Geometry: final body of the model. Coordinates: model frame, mm. A direction names the side the tool comes from. Coordinates: 2 decimals unless noted, no trailing zeros. Order: outer loops, then holes, each group sorted by start corner. A loop starts at its lowest first (then second) coordinate and runs counter-clockwise, first axis right, second up. Notation, with made-up numbers: M -33,-27.75 L -24,-27.75 A33 cw -24,5.25 Z; hole C -30.5,-14.5 d9. An arc over 180 degrees is marked long. Use CSV: the item, a comma, the result in double quotes. Start each with the question number.
1. Section query D-D on x = -47. Return the cut outline in (y, z).
2. Pull-direction query (X, two-part tool) for faces 1 (the flat face through (-52.798, 14, -26)), 2 (the cylindrical face through (50.149, 20.585, -26.644)), 3 (the cylindrical face through (45.193, 50.176, -15.773)), 4 (the flat face through (29, 32, -43.7)); classes: pulls with the +X half, pulls with the -X half, needs draft (parallel to the pull), parting line crosses it, or undercut.
3. First-contact query: P1, Ø11, axis at x = -24.5, z = 6, coming from the +Y side; P2, Ø10, axis at x = -30, z = -40.5, coming from the +Y side; P3, Ø4, axis at y = 37.5, z = -12.5, coming from the -X side. Flat tips, straight axial feed; report the tip coordinate or a pass-through.
4. Section query A-A on z = -32.5. Return the cut outline in (x, y), and give its area (3 significant figures).
5. Material intervals for line 1 (Z direction, x = 41, y = 49); line 2 (Y direction, x = 47, z = -19.5); line 3 (X direction, y = 10.5, z = -34), sorted ascending.
6. Set-up query: faces 5 (the flat face through (-6, 5, -34)), 6 (the flat face through (-37.798, 23, -26)), 7 (the flat face through (-36, 0, 4)). Return all of +Z, -Z, +X, -X, +Y, -Y with unobstructed straight access to the full face (end or side cutting, diameter ignored); none if empty.
7. Section query C-C on y = 87.45. Return the cut outline in (x, z), and give its area (4 significant figures).
8. Section query B-B on x = 47. Return the cut outline in (y, z).
from build123d import *

# Parameters (mm, degrees)
SKETCH2_W                      = 90
SKETCH2_H                      = 30
BOSS_EXTRUDE1_DEPTH            = 184.15
SHELL1_T                       = 8
FILLET1_R                      = 10
CUT_EXTRUDE1_DEPTH             = 15
BOSS_EXTRUDE3_DEPTH            = 12.7
SKETCH19_W                     = 50.7
SKETCH19_H                     = 190.15
CUT_EXTRUDE3_DEPTH             = 160
CUT_EXTRUDE4_DEPTH             = 62.424750712
CUT_EXTRUDE5_DEPTH             = 83.99843372
CUT_EXTRUDE5_DEPTH_BACK        = 83.99843372
SKETCH21_W                     = 50.7
SKETCH21_H                     = 2
SKETCH22_W                     = 105.595917942
SKETCH22_H                     = 28.653888285
BOSS_EXTRUDE4_DEPTH            = 18
SKETCH25_W                     = 12
SKETCH25_H                     = 6
CUT_EXTRUDE7_DEPTH             = 69.833963067
BOSS_EXTRUDE6_DEPTH            = 10
SKETCH27_W                     = 12
SKETCH27_H                     = 8
BOSS_EXTRUDE7_DEPTH            = 26
SKETCH31_W                     = 15
SKETCH31_H                     = 38.653888285
BOSS_EXTRUDE8_DEPTH            = 10
F_5_16_0_3125_DIAMETER_HOLE2_D = 7.9375
SKETCH35_W                     = 52.9
SKETCH35_H                     = 70.8
BOSS_EXTRUDE9_DEPTH            = 15
F_5_5_5_5_DIAMETER_HOLE1_D     = 5.5
BOSS_EXTRUDE10_DEPTH           = 38.653888285
CUT_EXTRUDE8_DEPTH             = 20
CUT_EXTRUDE10_DEPTH            = 2
SKETCH43_W                     = 14.246111715
SKETCH43_H                     = 10
CUT_EXTRUDE11_DEPTH            = 157.542244125


with BuildPart() as part:
    # Sketch2 → Boss-Extrude1 (new body)
    with BuildSketch(Plane(origin=(0, 0, 0), x_dir=(1, 0, 0), z_dir=(0, 1, 0))):
        Rectangle(SKETCH2_W, SKETCH2_H)
    extrude(amount=BOSS_EXTRUDE1_DEPTH)

    # Shell1
    shell1_openings = [part.faces().sort_by_distance(p)[0] for p in [
        (0, 92.075, 15),
    ]]
    offset(amount=SHELL1_T, openings=shell1_openings, kind=Kind.INTERSECTION)

    # Fillet1
    # the kernel refuses this fillet: 10 mm, written as the material it adds along each edge
    with BuildSketch(Plane(origin=(-45, 0, -15), x_dir=(0, 1, 0), z_dir=(0, 0, 1)), Plane(origin=(45, 0, 15), x_dir=(0, 1, 0), z_dir=(0, 0, -1))) as fillet1_piece_1:
        with BuildLine():
            CenterArc((FILLET1_R, -FILLET1_R), FILLET1_R, 90, 90)
            Line((0, -FILLET1_R), (0, 0))
            Line((0, 0), (FILLET1_R, 0))
        make_face()
    extrude(amount=30)
    with BuildSketch(Plane(origin=(-45, 184.15, -15), x_dir=(0, -1, 0), z_dir=(0, 0, 1)), Plane(origin=(45, 184.15, 15), x_dir=(0, -1, 0), z_dir=(0, 0, -1))) as fillet1_piece_2:
        with BuildLine():
            CenterArc((FILLET1_R, FILLET1_R), FILLET1_R, 180, 90)
            Line((0, FILLET1_R), (0, 0))
            Line((0, 0), (FILLET1_R, 0))
        make_face()
    extrude(amount=30)
    # the kernel refuses this fillet: 10 mm, written as the material it takes off along each edge
    with BuildSketch(Plane(origin=(53, 192.15, 40), x_dir=(0, -1, 0), z_dir=(0, 0, -1)), Plane(origin=(-53, 192.15, -48), x_dir=(0, -1, 0), z_dir=(0, 0, 1)), Plane(origin=(-53, -8, -48), x_dir=(1, 0, 0), z_dir=(0, 0, 1))) as fillet1_2_piece_1:
        with BuildLine():
            CenterArc((FILLET1_R, FILLET1_R), FILLET1_R, 180, 90)
            Line((0, FILLET1_R), (0, 0))
            Line((0, 0), (FILLET1_R, 0))
        make_face()
    extrude(amount=88, mode=Mode.SUBTRACT)
    with BuildSketch(Plane(origin=(53, -8, 40), x_dir=(0, 1, 0), z_dir=(0, 0, -1))) as fillet1_2_piece_2:
        with BuildLine():
            CenterArc((FILLET1_R, -FILLET1_R), FILLET1_R, 90, 90)
            Line((0, -FILLET1_R), (0, 0))
            Line((0, 0), (FILLET1_R, 0))
        make_face()
    extrude(amount=88, mode=Mode.SUBTRACT)

    # Sketch3 → Cut-Extrude1 (cut)
    with BuildSketch(Plane.XZ.offset(8)):
        with BuildLine():
            Line((-21.5, 15), (21.5, 15))
            Line((21.5, 15), (21.5, 0))
            ThreePointArc((21.5, 0), (16.888679541, -5.139118926), (10.252551286, -7.046111715))
            Line((10.252551286, -7.046111715), (-10.252551286, -7.046111715))
            ThreePointArc((-10.252551286, -7.046111715), (-16.888679541, -5.139118926), (-21.5, 0))
            Line((-21.5, 0), (-21.5, 15))
        make_face()
    extrude(amount=-CUT_EXTRUDE1_DEPTH, mode=Mode.SUBTRACT)

    # Sketch16 → Boss-Extrude3 (add)
    with BuildSketch(Plane(origin=(0, 0, -23), x_dir=(-1, 0, 0), z_dir=(0, 0, -1))):
        with BuildLine():
            Line((-53, 182.15), (-53, 2))
            ThreePointArc((-53, 2), (-50.071067812, -5.071067812), (-43, -8))
            Line((-43, -8), (43, -8))
            ThreePointArc((43, -8), (50.071067812, -5.071067812), (53, 2))
            Line((53, 2), (53, 182.15))
            ThreePointArc((53, 182.15), (50.071067812, 189.221067812), (43, 192.15))
            Line((43, 192.15), (-43, 192.15))
            ThreePointArc((-43, 192.15), (-50.071067812, 189.221067812), (-53, 182.15))
        make_face()
    extrude(amount=BOSS_EXTRUDE3_DEPTH)

    # Sketch19 → Cut-Extrude3 (cut)
    with BuildSketch(Plane(origin=(53, 0, 0), x_dir=(0, 0, -1), z_dir=(1, 0, 0))):
        with Locations((10.35, 97.075)):
            Rectangle(SKETCH19_W, SKETCH19_H)
    extrude(amount=-CUT_EXTRUDE3_DEPTH, mode=Mode.SUBTRACT)

    # Sketch20 → Cut-Extrude4 (cut, through all)
    with BuildSketch(Plane.XY.offset(-15)):
        with BuildLine():
            Line((41, 2), (-41, 2))
            ThreePointArc((-41, 2), (-38.16227766, 0.513167019), (-35, 0))
            Line((-35, 0), (35, 0))
            ThreePointArc((35, 0), (38.16227766, 0.513167019), (41, 2))
        make_face()
    extrude(amount=-CUT_EXTRUDE4_DEPTH, mode=Mode.SUBTRACT)

    # Sketch21 → Cut-Extrude5 (cut, two sides: drawn at the far end of the back side and taken through both)
    with BuildSketch(Plane.ZY.offset(-21.5).offset(-CUT_EXTRUDE5_DEPTH_BACK)):
        with Locations((-10.35, 1)):
            Rectangle(SKETCH21_W, SKETCH21_H)
    extrude(amount=CUT_EXTRUDE5_DEPTH + CUT_EXTRUDE5_DEPTH_BACK, mode=Mode.SUBTRACT)

    # Sketch22 → Boss-Extrude4 (add)
    with BuildSketch(Plane(origin=(0, 0, 0), x_dir=(1, 0, 0), z_dir=(0, 1, 0))):
        with Locations((0, 21.373055858)):
            Rectangle(SKETCH22_W, SKETCH22_H)
    extrude(amount=BOSS_EXTRUDE4_DEPTH)

    # Sketch25 → Cut-Extrude7 (cut, through all)
    with BuildSketch(Plane(origin=(0, 18, 0), x_dir=(1, 0, 0), z_dir=(0, 1, 0))):
        with Locations((0, 32.7)):
            Rectangle(SKETCH25_W, SKETCH25_H)
    extrude(amount=-CUT_EXTRUDE7_DEPTH, mode=Mode.SUBTRACT)

    # Sketch26 → Boss-Extrude6 (add)
    with BuildSketch(Plane(origin=(0, 0, -35.7), x_dir=(-1, 0, 0), z_dir=(0, 0, -1))):
        with BuildLine():
            Line((6, 18), (6, -8))
            Line((6, -8), (43, -8))
            ThreePointArc((43, -8), (49.32455532, -5.745966692), (52.797958971, 0))
            Line((52.797958971, 0), (52.797958971, 18))
            Line((52.797958971, 18), (6, 18))
        make_face()
        with BuildLine():
            Line((-6, -8), (-6, 18))
            Line((-6, 18), (-52.797958971, 18))
            Line((-52.797958971, 18), (-52.797958971, 0))
            ThreePointArc((-52.797958971, 0), (-49.32455532, -5.745966692), (-43, -8))
            Line((-43, -8), (-6, -8))
        make_face()
    extrude(amount=BOSS_EXTRUDE6_DEPTH)

    # Sketch27 → Boss-Extrude7 (add)
    with BuildSketch(Plane.XZ.offset(8)):
        with Locations((0, -41.7)):
            Rectangle(SKETCH27_W, SKETCH27_H)
    extrude(amount=-BOSS_EXTRUDE7_DEPTH)

    # Sketch31 → Boss-Extrude8 (add)
    with BuildSketch(Plane(origin=(0, 18, 0), x_dir=(1, 0, 0), z_dir=(0, 1, 0))):
        with Locations((-45.297958971, 26.373055858)):
            Rectangle(SKETCH31_W, SKETCH31_H)
        with Locations((45.297958971, 26.373055858)):
            Rectangle(SKETCH31_W, SKETCH31_H)
    extrude(amount=BOSS_EXTRUDE8_DEPTH)

    # 5/16 (0.3125) Diameter Hole2 (through all)
    with Locations(Plane.XY.offset(-7.046111715)):
        with Locations((-47, 23), (47, 23)):
            Hole(F_5_16_0_3125_DIAMETER_HOLE2_D / 2)

    # Sketch35 → Boss-Extrude9 (add)
    with BuildSketch(Plane(origin=(52.797958971, 0, 0), x_dir=(0, 0, -1), z_dir=(1, 0, 0))):
        with Locations((33.496111715, 63.4)):
            Rectangle(SKETCH35_W, SKETCH35_H)
    extrude(amount=-BOSS_EXTRUDE9_DEPTH)

    # Ø5.5 (5.5) Diameter Hole1 (through all)
    with Locations(Plane(origin=(52.797958971, 0, 0), x_dir=(0, 0, -1), z_dir=(1, 0, 0))):
        with Locations((48.596111715, 87.45), (18.396111715, 87.45), (18.396111715, 49.35), (48.596111715, 49.35)):
            Hole(F_5_5_5_5_DIAMETER_HOLE1_D / 2)

    # Sketch39 → Boss-Extrude10 (add)
    with BuildSketch(Plane.XY.offset(-7.046111715)):
        Polygon((7.797958971, 18), (37.797958971, 18), (37.797958971, 68), align=None)
    extrude(amount=-BOSS_EXTRUDE10_DEPTH)

    # Sketch40 → Cut-Extrude8 (cut)
    with BuildSketch(Plane.XY.offset(-7.046111715)):
        Polygon((37.797958971, 68), (7.797958971, 18), (37.797958971, 18), align=None)
    extrude(amount=-CUT_EXTRUDE8_DEPTH, mode=Mode.SUBTRACT)

    # Sketch42 → Cut-Extrude10 (cut)
    with BuildSketch(Plane(origin=(0, 0, -45.7), x_dir=(-1, 0, 0), z_dir=(0, 0, -1))):
        Polygon((-37.797958971, 68), (-7.797958971, 18), (-37.797958971, 18), align=None)
    extrude(amount=-CUT_EXTRUDE10_DEPTH, mode=Mode.SUBTRACT)

    # Sketch43 → Cut-Extrude11 (cut, through all)
    with BuildSketch(Plane(origin=(52.797958971, 0, 0), x_dir=(0, 0, -1), z_dir=(1, 0, 0))):
        with Locations((52.823055858, 33)):
            Rectangle(SKETCH43_W, SKETCH43_H)
    extrude(amount=-CUT_EXTRUDE11_DEPTH, mode=Mode.SUBTRACT)


solid = part.part
Results list:
1,outline,"M -7.17,-45.7 L 19.03,-45.7 L 19.03,-7.05 L 0,-7.05 L 0,15 L -7.17,15 Z; M 26.97,-45.7 L 28,-45.7 L 28,-7.05 L 26.97,-7.05 Z"
2,face 1,"pulls with the -X half"
2,face 2,"undercut"
2,face 3,"needs draft"
2,face 4,"undercut"
3,P1,"stops at y = 0"
3,P2,"stops at y = 18"
3,P3,"stops at x = 37.8"
4,outline,"M -52.8,0 A10 ccw -43,-8 L -6,-8 L -6,18 L -37.8,18 L -37.8,28 L -52.8,28 Z; M 6,-8 L 43,-8 A10 ccw 52.8,0 L 52.8,98.8 L 37.8,98.8 L 37.8,68 L 7.8,18 L 6,18 Z; hole C -47,23 d7.94; hole C 47,23 d7.94"
4,area,"4,410 mm²"
5,line 1,"z = -59.95 to -51.32, -45.87 to -21.12, -15.67 to -7.05"
5,line 2,"y = -7.17 to 19.03, 26.97 to 46.83, 51.87 to 84.93, 89.97 to 98.8"
5,line 3,"x = -52.8 to -6, 6 to 52.8"
6,face 5,"+Y, -Y"
6,face 6,"+Z, -Z, +Y"
6,face 7,"+Z, +X, -X, +Y"
7,outline,"M 37.8,-59.95 L 52.8,-59.95 L 52.8,-51.35 L 37.8,-51.35 Z; M 37.8,-45.85 L 52.8,-45.85 L 52.8,-21.15 L 37.8,-21.15 Z; M 37.8,-15.65 L 52.8,-15.65 L 52.8,-7.05 L 37.8,-7.05 Z"
7,area,"628.5 mm²"
8,outline,"M -7.17,-45.7 L 19.03,-45.7 L 19.03,-7.05 L 0,-7.05 L 0,15 L -7.17,15 Z; M 26.97,-45.7 L 38,-45.7 L 38,-59.95 L 98.8,-59.95 L 98.8,-7.05 L 26.97,-7.05 Z; hole C 49.35,-48.6 d5.5; hole C 49.35,-18.4 d5.5; hole C 87.45,-48.6 d5.5; hole C 87.45,-18.4 d5.5"
